from build123d import *

# Parameters (mm, degrees)
BOSS_EXTRUDE2_DEPTH = 6.35
SHELL3_T            = -1.27
SKETCH2_7_R         = 4.7625
SKETCH2_7_R_2       = 3.175
CUT_EXTRUDE2_DEPTH  = 30.315069184
BOSS_EXTRUDE3_DEPTH = 1.524
CUT_EXTRUDE3_REACH  = 34.391


with BuildPart() as part:
    # Sketch2 → Boss-Extrude2 (new body)
    with BuildSketch(Plane(origin=(0, 0, 0), x_dir=(0, 1, 0), z_dir=(0, 0, 1))):
        with BuildLine():
            Line((8.659090909, -13.305478933), (20.926136364, -5.322191573))
            ThreePointArc((20.926136364, -5.322191573), (23.8125, 0), (20.926136364, 5.322191573))
            Line((20.926136364, 5.322191573), (8.659090909, 13.305478933))
            ThreePointArc((8.659090909, 13.305478933), (-15.875, 0), (8.659090909, -13.305478933))
        make_face()
    extrude(amount=BOSS_EXTRUDE2_DEPTH)

    # Shell3
    shell3_openings = [part.faces().sort_by_distance(p)[0] for p in [
        (0, 2.303090429, 6.35),
    ]]
    offset(amount=SHELL3_T, openings=shell3_openings, kind=Kind.INTERSECTION)

    # Sketch2_7 → Cut-Extrude2 (cut, through all)
    with BuildSketch(Plane(origin=(0, 0, 0), x_dir=(0, 1, 0), z_dir=(0, 0, 1))):
        with Locations(Location((0, 0, 0), (0, 0, 270))):
            Circle(SKETCH2_7_R)
        with Locations(Location((17.4625, 0, 0), (0, 0, 270))):
            Circle(SKETCH2_7_R_2)
    extrude(amount=CUT_EXTRUDE2_DEPTH, mode=Mode.SUBTRACT)

    # Sketch6 → Boss-Extrude3 (add)
    with BuildSketch(Plane(origin=(0, 0, 5.715), x_dir=(0, -1, 0), z_dir=(0, 0, 1))):
        Polygon((-16.423409091, 8.252527639), (-17.4625, 9.849185111), (-14.269185056, 11.927366929), (-13.230094147, 10.330709457), align=None)
        Polygon((-14.269185056, -11.927366929), (-13.230094147, -10.330709457), (-16.423409091, -8.252527639), (-17.4625, -9.849185111), align=None)
    extrude(amount=BOSS_EXTRUDE3_DEPTH)

    # Sketch8 → Cut-Extrude3 (cut, up to next)
    with BuildSketch(Plane(origin=(-5.052951293, 7.764318182, 0), x_dir=(-0.8381404052084441, -0.5454545454545457, 0), z_dir=(-0.5454545454545457, 0.8381404052084441, 0)), mode=Mode.PRIVATE) as cut_extrude3_sk1:
        Polygon((-17.272, 6.985), (-17.018, 6.985), (-17.018, 7.239), (-15.875, 7.239), (-15.875, 6.35), (-15.875, 6.096), (-17.272, 6.096), align=None)
    cut_extrude3_tool1 = extrude(cut_extrude3_sk1.sketch, amount=-CUT_EXTRUDE3_REACH, mode=Mode.PRIVATE) & part.part
    cut_extrude3 = cut_extrude3_tool1.solids().sort_by_distance((8.8178, 16.791284, 6.648784))[0]
    add(cut_extrude3, mode=Mode.SUBTRACT)

    # Mirror1: Cut-Extrude3 across plane
    add(cut_extrude3.mirror(Plane(origin=(0, 0, 0), x_dir=(0, 0, 1), z_dir=(1, 0, 0))), mode=Mode.SUBTRACT)


solid = part.part
Build history of the part. All positions in model axes, mm. A direction names the side the tool comes from. Round coordinates to 2 decimals unless told otherwise and drop trailing zeros. One line per item, written item: value. Start each with the question number.
Q1. Drop flat-ended pins along their axis: pin 1 Ø1 at (x, z) = (-0.5, 6.5) entering from +Y; pin 2 Ø7.5 at (x, y) = (0, 17.46) entering from +Z; pin 3 Ø3 at (y, z) = (19.5, 3) entering from -X; pin 4 Ø1.8 at (x, y) = (-10.5, 15) entering from -Z (3 decimals). Give the stop position or say it passes through.
Q2. 3-axis set-ups, long thin cutter, end or side, ignore diameter. For faces 5 (the face through (-11.67, 14.1, 6.3)), 6 (the face through (3, 4, 1.27)), 7 (the face through (11.67, 14.1, 6.3)), 8 (the face through (-9.6, 17.3, 6.3)), 9 (the face through (-10, 15, 5.715)): which of +Z, -Z, +X, -X, +Y, -Y reach the whole face in a straight line?
Q3. Two-plate mould, pull along Y, no slides. Class faces 1 (the face through (9.6, 17.3, 6.3)), 2 (the face through (-8.19, 14.19, 3.77)), 3 (the face through (-10.5, 15.7, 7.239)), 4 (the face through (-10, 15, 6.096)): released by +Y, released by -Y, zero draft, split by the parting line, or undercut.
Q4. Probe line 1 along Y through (x, z) = (0, 0.45) (1 decimal); line 2 along Y through (x, z) = (0, 5.5) (1 decimal); line 3 along X through (y, z) = (0, 0.4) (1 decimal). List the from-to ranges inside material, lowest first.
Q5. Cut at A-A on x = 0. Count the separate pieces of the cut face and the enclosed holes in it, plus the area to 3 significant figures.
Computed:
1. pin 1: y = 23.81
1. pin 2: z = 1.27
1. pin 3: x = -7.23
1. pin 4: z = 5.715
2. face 5: +Z, -Z, -X
2. face 6: +Z
2. face 7: +Z, -Z, +X
2. face 8: +Z, -Z, +Y
2. face 9: -Z, -X, +Y
3. face 1: released by +Y
3. face 2: undercut
3. face 3: zero draft
3. face 4: undercut
4. line 1: -15.9 to -4.8, 4.8 to 14.3, 20.6 to 23.8
4. line 2: -15.9 to -14.6, 22.5 to 23.8
4. line 3: -15.9 to -4.8, 4.8 to 15.9
5. separate pieces: 3
5. enclosed holes: 0
5. area: 43.1 mm²
